Read the model definition and answer for the solid it produces. Units are mm, in the model's axes. Coordinates: 2 decimals unless noted, no trailing zeros. Loops run counter-clockwise (first coordinate to the right, second up) from the corner with the lowest first, then second, coordinate; pieces in that order, holes last.
from build123d import *

# Parameters (mm, degrees)
F0_R          = 8
F0_R_2        = 2.5
F1_DEPTH      = 2.5
F1_DEPTH_BACK = 2.5
F2_R          = 6.9
F2_R_2        = 4.5
F3_DEPTH      = 0.1


# Not quite as in the source:
# - a pattern or mirror of a feature is missing from the dataset's text; its kind, count and spacing are read off the source's solid


with BuildPart() as f1:
    # F0 (on Right) → F1 (new body, two sides)
    with BuildSketch(Plane.YZ) as f1_sk:
        Circle(F0_R)
        Circle(F0_R_2, mode=Mode.SUBTRACT)
    extrude(amount=F1_DEPTH)
    extrude(f1_sk.sketch, amount=-F1_DEPTH_BACK)

    # F2 (on face) → F3 (cut)
    with BuildSketch(Plane.YZ.offset(2.5)):
        Circle(F2_R)
        Circle(F2_R_2, mode=Mode.SUBTRACT)
    f3 = extrude(amount=-F3_DEPTH, mode=Mode.SUBTRACT)

    # F3_copies: F3 across plane
    add(f3.mirror(Plane(origin=(0, 0, 0), x_dir=(0, 0, -1), z_dir=(-1, 0, 0))), mode=Mode.SUBTRACT)


solid = f1.part
Q1. A cutting plane is placed at A-A (z = 0). Give the vertices of the cut face in (x, y).
Findings below:
outline: (-2.5, -8) - (2.5, -8) - (2.5, -6.9) - (2.4, -6.9) - (2.4, -4.5) - (2.5, -4.5) - (2.5, -2.5) - (-2.5, -2.5) - (-2.5, -4.5) - (-2.4, -4.5) - (-2.4, -6.9) - (-2.5, -6.9) - close; (-2.5, 2.5) - (2.5, 2.5) - (2.5, 4.5) - (2.4, 4.5) - (2.4, 6.9) - (2.5, 6.9) - (2.5, 8) - (-2.5, 8) - (-2.5, 6.9) - (-2.4, 6.9) - (-2.4, 4.5) - (-2.5, 4.5) - close
Q2. Straight lines are drawn through the part: probe 1 along Z at (x, y) = (1.25, 0); probe 2 along X at (y, z) = (-3.75, -3.75); probe 3 along Z at (x, y) = (1.75, 0.5). For each, find the intervals that lie inside material, in ascending order.
Findings below:
probe 1: z = -8 to -2.5, 2.5 to 8
probe 2: x = -2.4 to 2.4
probe 3: z = -7.98 to -2.45, 2.45 to 7.98
Q3. Flat-ended cylindrical pins translate along their axes: pin 1 Ø2 at (x, y) = (-0.5, -0.5) entering from +Z; pin 2 Ø1 at (x, z) = (-1, 1.5) entering from -Y. Find the tip coordinate at first contact, or state that the pin passes through.
Findings below:
pin 1: stops at z = 8
pin 2: stops at y = -7.94
Q4. Determine the mould class of faces 1 (the face through (0.04, -1.73, -7.81)), 2 (the face through (2.5, 2, -2)), 3 (the face through (2.4, 0, -5)), 4 (the face through (-2.4, 0, -5)) for opening direction Y: +Y half, -Y half, draft (parallel to the pull), parting line (faces both ways), or undercut.
Findings below:
face 1: parting line
face 2: draft
face 3: undercut
face 4: undercut
Q5. A cutting plane is placed at D-D (x = 1.4). Give the vertices of the cut face in (y, z), then the cut area to 3 significant figures.
Findings below:
outline: circle Ø16 at (0, 0); hole circle Ø5 at (0, 0)
area: 181 mm2
Q6. A cutting plane is placed at C-C (z = -6). Give the vertices of the cut face in (x, y), then the cut area to 3 significant figures.
Findings below:
outline: (-2.5, -5.29) - (2.5, -5.29) - (2.5, -3.41) - (2.4, -3.41) - (2.4, 3.41) - (2.5, 3.41) - (2.5, 5.29) - (-2.5, 5.29) - (-2.5, 3.41) - (-2.4, 3.41) - (-2.4, -3.41) - (-2.5, -3.41) - close
area: 51.6 mm2
